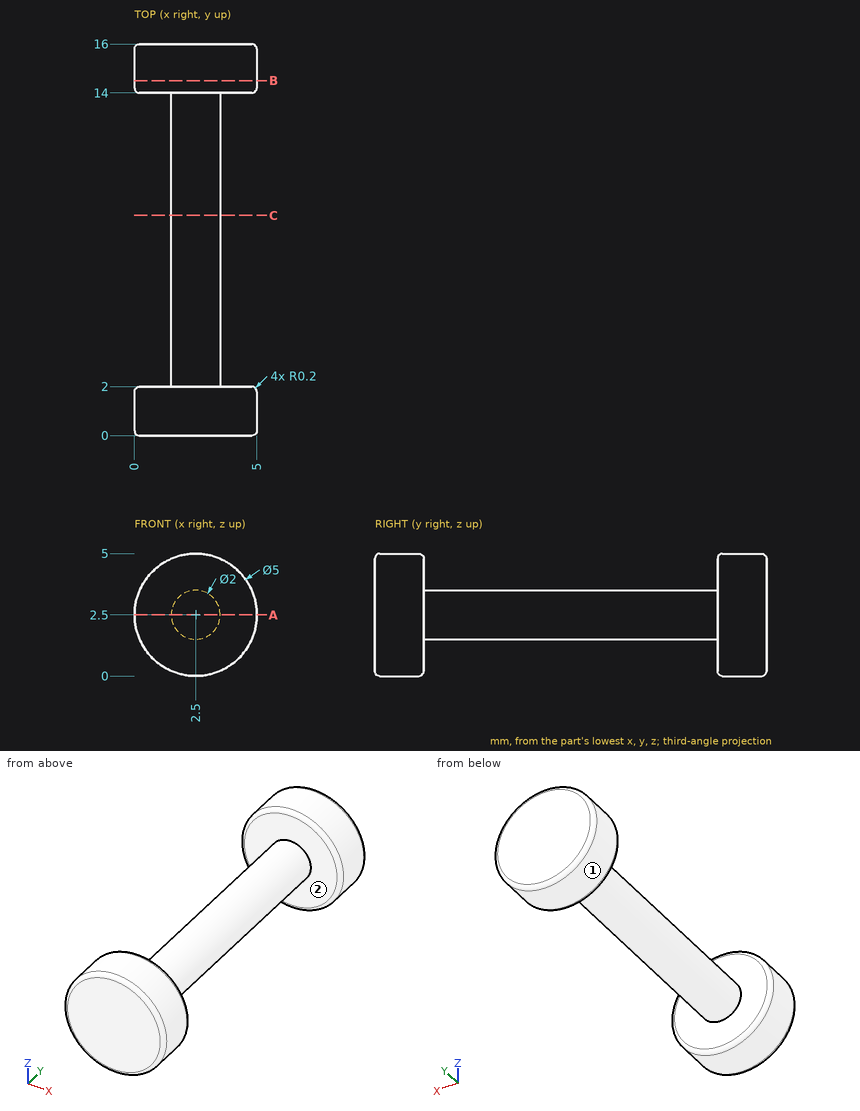
Answer from the drawing. Dimensions are ordinates in mm from the lowest x, y and z of the part. A direction names the side the tool comes from. Coordinates: 2 decimals unless noted, no trailing zeros. Write each loop counter-clockwise with the first axis right and the second up, starting at its lowest first coordinate (ties: lowest second). Pieces come first, ordered by that corner, then holes. Notation, with made-up numbers: M 2,30 L 27,30 A18 cw 27,61 Z; hole C 47,-36.75 d10. An arc over 180 degrees is marked long. Use one line per item in the form item = value. Start each with the question number.
1. The part is cut by section A-A (z = 2.5). Give the vertices of the cut face in (x, y), plus the area to 3 significant figures.
2. A tool of negligible diameter and unlimited length cuts with its end or side. For the marked faces 1 and 2, from which of +Z, -Z, +X, -X, +Y, -Y can it reach the whole face along a straight path? Write none if from no direction.
3. The part is cut by section B-B (y = 14.5). Give the vertices of the cut face in (x, z), plus the area to 3 significant figures.
4. Straight lines are drawn through the part: probe 1 along Y at (x, z) = (2, 4.5); probe 2 along Z at (x, y) = (2.6, 15); probe 3 along Z at (x, y) = (2.5, 6). For each, find the intervals that lie inside material, in ascending order. Write a range as from..to.
5. Each of these flat-tipped pins is pushed along its axis until it touches: P1, Ø3, axis at x = 4.5, y = 3, coming from the +Z side; P2, Ø3, axis at x = 0.5, y = 13.5, coming from the -Z side. Where does it stop, or does it pass through?
6. The part is cut by section C-C (y = 9). Give the vertices of the cut face in (x, z).
Evaluation:
q1.outline = M 0,0.2 A0.2 ccw 0.2,0 L 4.8,0 A0.2 ccw 5,0.2 L 5,1.8 A0.2 ccw 4.8,2 L 3.5,2 L 3.5,14 L 4.8,14 A0.2 ccw 5,14.2 L 5,15.8 A0.2 ccw 4.8,16 L 0.2,16 A0.2 ccw 0,15.8 L 0,14.2 A0.2 ccw 0.2,14 L 1.5,14 L 1.5,2 L 0.2,2 A0.2 ccw 0,1.8 Z
q1.area = 43.9 mm^2
q2.face_1 = +Y, -Y
q2.face_2 = none
q3.outline = C 2.5,2.5 d5
q3.area = 19.6 mm^2
q4.probe_1 = 0..2, 14..16
q4.probe_2 = 0..5
q4.probe_3 = 1.5..3.5
q5.P1 = 4.77
q5.P2 = 0.09
q6.outline = C 2.5,2.5 d2
